```python
from build123d import *

# Parameters (mm, degrees)
BOSS_EXTRUDE1_DEPTH = 15.3
SKETCH4_W           = 7
SKETCH4_H           = 5.9
CUT_EXTRUDE1_DEPTH  = 78.461901488
SKETCH5_W           = 74.8
SKETCH5_H           = 19.8
BOSS_EXTRUDE2_DEPTH = 2
SKETCH6_W           = 74.8
SKETCH6_H           = 3
BOSS_EXTRUDE3_DEPTH = 37.2
SKETCH7_W           = 37.2
SKETCH7_H           = 3
BOSS_EXTRUDE4_DEPTH = 5
FILLET1_R           = 3
BOSS_EXTRUDE5_DEPTH = 23.3
FILLET2_R           = 2
SKETCH10_W          = 74.8
SKETCH10_H          = 19.8
CUT_EXTRUDE2_DEPTH  = 0.2
CUT_EXTRUDE3_DEPTH  = 5
CUT_EXTRUDE3_DRAFT  = 30
BOSS_EXTRUDE6_DEPTH = 15
CUT_EXTRUDE4_START  = -80.1
SKETCH15_W          = 92.424256673
SKETCH15_H          = 46.662169566
CUT_EXTRUDE4_DEPTH  = 80.1


with BuildPart() as part:
    # Sketch1 → Boss-Extrude1 (new body)
    with BuildSketch(Plane(origin=(0, 0, 0), x_dir=(1, 0, 0), z_dir=(0, 1, 0))):
        with BuildLine():
            Line((1.005677457, 13.08496015), (1.005677457, -6.71503985))
            Line((1.005677457, -6.71503985), (10.705677457, -6.71503985))
            Line((10.705677457, -6.71503985), (10.705677457, 7.68496015))
            ThreePointArc((10.705677457, 7.68496015), (24.690281417, 4.453424809), (33.705677457, -6.71503985))
            Line((33.705677457, -6.71503985), (75.805677457, -6.71503985))
            Line((75.805677457, -6.71503985), (75.805677457, 13.08496015))
            Line((75.805677457, 13.08496015), (1.005677457, 13.08496015))
        make_face()
    extrude(amount=BOSS_EXTRUDE1_DEPTH)

    # Sketch4 → Cut-Extrude1 (cut, through all)
    with BuildSketch(Plane(origin=(75.805677457, 0, 0), x_dir=(0, 0, -1), z_dir=(1, 0, 0))):
        with Locations((-3.21503985, 7.3)):
            Rectangle(SKETCH4_W, SKETCH4_H)
    extrude(amount=-CUT_EXTRUDE1_DEPTH, mode=Mode.SUBTRACT)

    # Sketch5 → Boss-Extrude2 (add)
    with BuildSketch(Plane(origin=(0, 15.3, 0), x_dir=(1, 0, 0), z_dir=(0, 1, 0))):
        with Locations((38.405677457, 3.18496015)):
            Rectangle(SKETCH5_W, SKETCH5_H)
    extrude(amount=BOSS_EXTRUDE2_DEPTH)

    # Sketch6 → Boss-Extrude3 (add)
    with BuildSketch(Plane(origin=(0, 0, -13.08496015), x_dir=(-1, 0, 0), z_dir=(0, 0, -1))):
        with Locations((-38.405677457, 18.8)):
            Rectangle(SKETCH6_W, SKETCH6_H)
    extrude(amount=-BOSS_EXTRUDE3_DEPTH)

    # Sketch7 → Boss-Extrude4 (add)
    with BuildSketch(Plane.ZY.offset(-1.005677457)):
        with Locations((5.51503985, 18.8)):
            Rectangle(SKETCH7_W, SKETCH7_H)
    extrude(amount=BOSS_EXTRUDE4_DEPTH)

    # Fillet1
    fillet1_edges = [part.edges().sort_by_distance(p)[0] for p in [
        (-3.994322543, 18.8, 24.11503985),
    ]]
    fillet(fillet1_edges, radius=FILLET1_R)

    # Sketch8 → Boss-Extrude5 (add)
    with BuildSketch(Plane(origin=(0, 20.3, 0), x_dir=(1, 0, 0), z_dir=(0, 1, 0))):
        with BuildLine():
            Line((75.805677457, 13.08496015), (90.805677457, 13.08496015))
            Line((90.805677457, 13.08496015), (90.805677457, -3.072659154))
            ThreePointArc((90.805677457, -3.072659154), (86.671822493, -15.993396221), (75.805677457, -24.11503985))
            Line((75.805677457, -24.11503985), (75.805677457, 13.08496015))
        make_face()
    extrude(amount=-BOSS_EXTRUDE5_DEPTH)

    # Fillet2
    fillet2_edges = [part.edges().sort_by_distance(p)[0] for p in [
        (90.805677457, -3, -5.006150498),
        (86.671822493, -3, 15.993396221),
    ]]
    fillet(fillet2_edges, radius=FILLET2_R)

    # Sketch10 → Cut-Extrude2 (cut)
    with BuildSketch(Plane(origin=(0, 0, 0), x_dir=(-1, 0, 0), z_dir=(0, -1, 0))):
        with Locations((-38.405677457, 3.18496015)):
            Rectangle(SKETCH10_W, SKETCH10_H)
    extrude(amount=-CUT_EXTRUDE2_DEPTH, mode=Mode.SUBTRACT)


with BuildPart() as cut_extrude3_tool:
    # Sketch11 → Cut-Extrude3 (with draft: the straight prism first)
    with BuildSketch(Plane(origin=(0, -3, 0), x_dir=(-1, 0, 0), z_dir=(0, -1, 0))):
        with BuildLine():
            Line((-75.805677457, 13.08496015), (-83.305677457, 13.08496015))
            Line((-83.305677457, 13.08496015), (-83.305677457, 8.08496015))
            ThreePointArc((-83.305677457, 8.08496015), (-80.312616551, 4.449551508), (-75.805677457, 3.08496015))
            Line((-75.805677457, 3.08496015), (-75.805677457, 13.08496015))
        make_face()
    extrude(amount=-CUT_EXTRUDE3_DEPTH)
    # Cut-Extrude3: the draft: its side faces are tilted about the plane it starts from
    cut_extrude3_sides = [cut_extrude3_tool.faces().sort_by_distance(p)[0] for p in [
        (75.805677457, -0.5, -8.08496015),
        (79.555677457, -0.5, -13.08496015),
        (83.305677457, -0.5, -10.58496015),
        (80.312616551, -0.5, -4.449551508),
    ]]
    draft(cut_extrude3_sides, Plane(origin=(0, -3, 0), x_dir=(-1, 0, 0), z_dir=(0, -1, 0)), CUT_EXTRUDE3_DRAFT)


with BuildPart() as part_1:
    add(part.part)

    # Cut-Extrude3: cut by cut_extrude3_tool
    add(cut_extrude3_tool.part, mode=Mode.SUBTRACT)

    # Sketch14 → Boss-Extrude6 (add)
    with BuildSketch(Plane(origin=(0, 0, -13.08496015), x_dir=(-1, 0, 0), z_dir=(0, 0, -1))):
        Polygon((-72.918926111, 2), (-73.958156595, 0.2), (-75.805677457, 0.2), (-75.805677457, 2), align=None)
    extrude(amount=-BOSS_EXTRUDE6_DEPTH)

    # Mirror1: part across plane


with BuildPart() as part_2:
    add(part_1.part)
    add(part_1.part.mirror(Plane(origin=(0, 15.3, -13.08496015), x_dir=(1, 0, 0), z_dir=(0, 0, -1))))

    # Sketch15 → Cut-Extrude4 (cut)
    with BuildSketch(Plane(origin=(90.805677457, 0, 0), x_dir=(0, 0, -1), z_dir=(1, 0, 0)).offset(CUT_EXTRUDE4_START)):
        with Locations((15.406225438, 7.825251121)):
            Rectangle(SKETCH15_W, SKETCH15_H)
    extrude(amount=CUT_EXTRUDE4_DEPTH, mode=Mode.SUBTRACT)


solid = part_2.part
```
Geometry: final body of the model. Coordinates: model frame, mm. A direction names the side the tool comes from. Round coordinates to 2 decimals unless told otherwise and drop trailing zeros. Order: outer loops, then holes, each group sorted by start corner. A loop starts at its lowest first (then second) coordinate and runs counter-clockwise, first axis right, second up. Notation, with made-up numbers: (-16.75, 85.25) -> (5.25, 85.25) arc R27 ccw to (5.25, 109.25) -> close; hole circle Ø2 at (40, 40.25). An arc over 180 degrees is marked (long way). Write each question's results on one line, items separated by ' | '.
Q1. Section query C-C (z = -17). Output: boundary loops of the cut face in (x, y), and give its area (3 significant figures).
Response values:
outline: (-3.99, 17.3) -> (1.01, 17.3) -> (1.01, 0.2) -> (10.71, 0.2) -> (10.71, 20.3) -> (-3.99, 20.3) -> close | area: 210 mm²
Q2. Ray query, line 1 along Y through (x, z) = (4, 0); line 2 along Y through (x, z) = (-1.5, -10); line 3 along Z through (x, y) = (3.5, 7.5). Return the intervals inside material, ascending.
Response values:
line 1: 0.2 to 4.35, 10.25 to 20.3 | line 2: 17.3 to 20.3 | line 3: -25.88 to -0.28
Q3. Pull-direction query (Y, two-part tool) for faces 1 (the face through (6, 4.35, 3)), 2 (the face through (6, 0.2, -13)), 3 (the face through (6, 7, -25.885)), 4 (the face through (6, 2, 6.715)); classes: released by +Y, released by -Y, zero draft, split by the parting line, or undercut.
Response values:
face 1: undercut | face 2: released by -Y | face 3: undercut | face 4: zero draft
Q4. Section query B-B (x = 5.5). Output: boundary loops of the cut face in (y, z), and give its area (3 significant figures).
Response values:
outline: (0.2, -32.88) -> (4.35, -32.88) -> (4.35, -25.88) -> (10.25, -25.88) -> (10.25, -32.88) -> (17.3, -32.88) -> (17.3, -50.28) -> (20.3, -50.28) -> (20.3, 24.12) -> (17.3, 24.12) -> (17.3, 6.72) -> (10.25, 6.72) -> (10.25, -0.28) -> (4.35, -0.28) -> (4.35, 6.72) -> (0.2, 6.72) -> close | area: 818 mm²
Q5. Section query A-A (z = 4). Output: boundary loops of the cut face in (x, y), and give its area (3 significant figures).
Response values:
outline: (-3.99, 17.3) -> (1.01, 17.3) -> (1.01, 10.25) -> (10.71, 10.25) -> (10.71, 20.3) -> (-3.99, 20.3) -> close; (1.01, 0.2) -> (10.71, 0.2) -> (10.71, 4.35) -> (1.01, 4.35) -> close | area: 153 mm²
Q6. Access query for faces 5 (the face through (1.006, 9, -13)), 6 (the face through (6, 10.25, -29)), 7 (the face through (6, 2, -32.885)). Directions: +Z, -Z, +X, -X, +Y, -Y. A direction counts if a zero-diameter tool reaches every point of the face in a straight line with its end or side. Return the directions, or none.
Response values:
face 5: +Z, -Z, -X, -Y | face 6: -Z, +X, -X | face 7: -Z, +X, -X, -Y
Q7. Section query D-D (y = 14.5). Output: boundary loops of the cut face in (x, z), and give its area (3 significant figures).
Response values:
outline: (1.01, -32.88) -> (10.71, -32.88) -> (10.71, 6.72) -> (1.01, 6.72) -> close | area: 384 mm²
Q8. Pin query (flat end, axial travel): pin 1 Ø3.5 at (x, y) = (6.5, 3.5) entering from -Z; pin 2 Ø5.5 at (x, y) = (3.5, 13) entering from +Z; pin 3 Ø3 at (x, z) = (-1, -8) entering from -Y. Return the tip coordinate at first contact, or that it passes through.
Response values:
pin 1: z = -32.88 | pin 2: z = 6.72 | pin 3: y = 17.3
